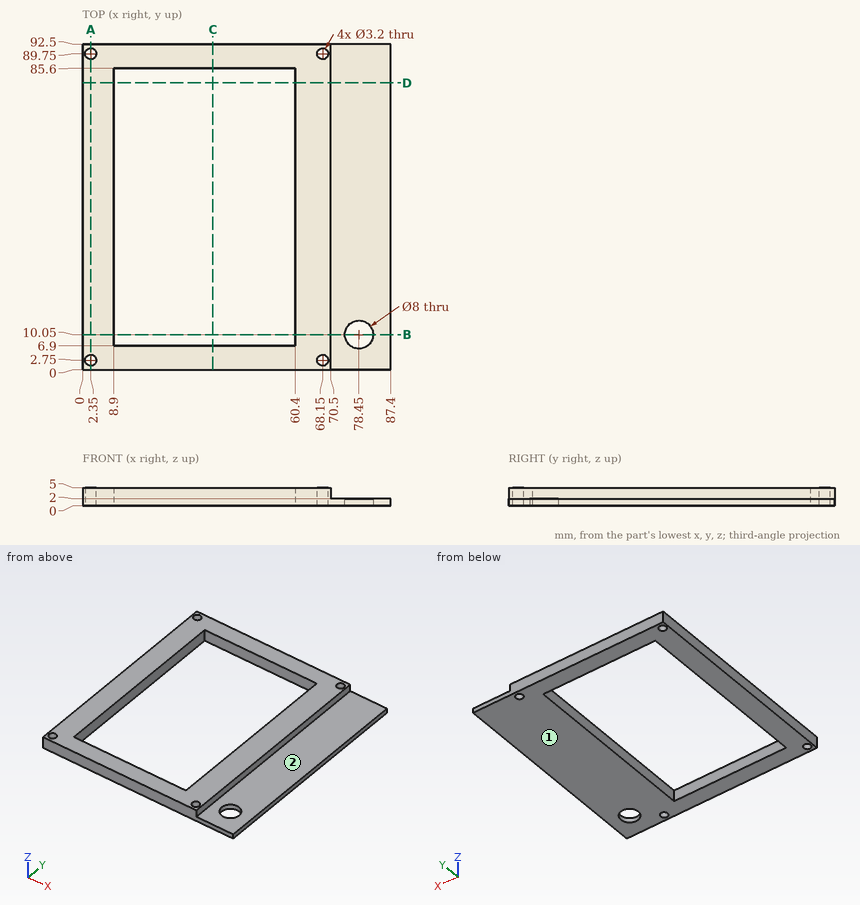
For this review, use the dimensioned drawing (mm, ordinates from the lowest corner) and the shaded views. A direction names the side the tool comes from. Give positions to 0.01 mm unless a question says otherwise; leave off trailing zeros. Loops run counter-clockwise (first coordinate to the right, second up) from the corner with the lowest first, then second, coordinate; pieces in that order, holes last. Notation, with made-up numbers: (71, 72) - (101, 72) arc R11 cw to (101, 76) - close; hole circle Ø1 at (-7, 87.25). An arc over 180 degrees is marked (long way). Write each question's results on one line, items separated by ' | '.
(1) Take a section at B-B (y = 10.05). Give the boundary of the cut face in (x, z).
Conclusion:
outline: (0, 0) - (8.9, 0) - (8.9, 5) - (0, 5) - close; (60.4, 0) - (74.45, 0) - (74.45, 2) - (70.5, 2) - (70.5, 5) - (60.4, 5) - close; (82.45, 0) - (87.4, 0) - (87.4, 2) - (82.45, 2) - close
(2) Take a section at D-D (y = 81.5). Give the boundary of the cut face in (x, z).
Conclusion:
outline: (0, 0) - (8.9, 0) - (8.9, 5) - (0, 5) - close; (60.4, 0) - (87.4, 0) - (87.4, 2) - (70.5, 2) - (70.5, 5) - (60.4, 5) - close
(3) Take a section at A-A (x = 2.35). Give the boundary of the cut face in (y, z), then the cut area to 4 significant figures.
Conclusion:
outline: (0, 0) - (1.15, 0) - (1.15, 5) - (0, 5) - close; (4.35, 0) - (88.15, 0) - (88.15, 5) - (4.35, 5) - close; (91.35, 0) - (92.5, 0) - (92.5, 5) - (91.35, 5) - close | area: 430.5 mm^2
(4) For pin 1 Ø0.9 at (y, z) = (26.5, 4) entering from +X; pin 2 Ø6.5 at (x, y) = (78.45, 10.05) entering from +Z; pin 3 Ø5 at (x, y) = (80.5, 53.5) entering from +Z, all flat-tipped, find the tip position at first contact; note any pin that passes through.
Conclusion:
pin 1: x = 70.5 | pin 2: through | pin 3: z = 2
(5) For the marked faces 1 and 2, list the 3-axis set-ups (+Z, -Z, +X, -X, +Y, -Y) from which the entire face can be reached by the end or side of a thin tool; tool diameter is ignored.
Conclusion:
face 1: -Z, +X, -X, +Y, -Y | face 2: +Z, +X, +Y, -Y
(6) Take a section at C-C (x = 37). Give the boundary of the cut face in (y, z).
Conclusion:
outline: (0, 0) - (6.9, 0) - (6.9, 5) - (0, 5) - close; (85.6, 0) - (92.5, 0) - (92.5, 5) - (85.6, 5) - close
(7) For line 1 along X through (y, z) = (89.75, 2.5); line 2 along Y through (x, z) = (2.35, 1.5); line 3 along X through (y, z) = (71.5, 3.75), list the stretches that pass through material, from the lowest coordinate up.
Conclusion:
line 1: 0 to 0.75, 3.95 to 66.55, 69.75 to 70.5 | line 2: 0 to 1.15, 4.35 to 88.15, 91.35 to 92.5 | line 3: 0 to 8.9, 60.4 to 70.5
